Can you work these out from the model? Positions are in its coordinate system, mm. Face numbers are marked on the shaded views. Give positions to 0.01 mm unless a question says otherwise; leave off trailing zeros. Loops run counter-clockwise (first coordinate to the right, second up) from the corner with the lowest first, then second, coordinate; pieces in that order, holes last. Notation, with made-up numbers: M 26,55.5 L 78,55.5 A15 ccw 78,68.5 Z; hole C 70,-33.75 d1. An arc over 180 degrees is marked long. One line per item, written item: value. Start each with the question number.
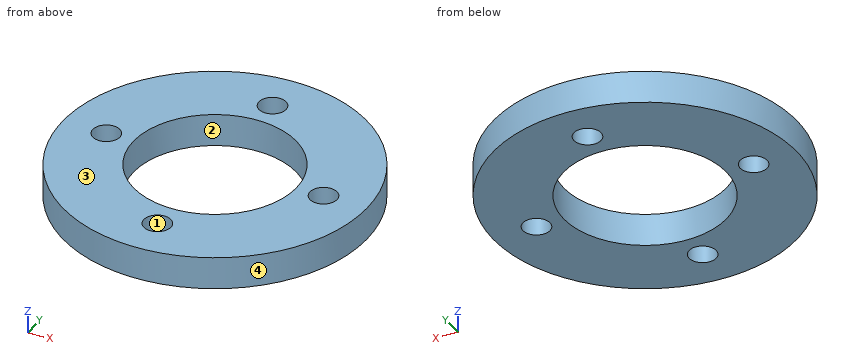
from build123d import *

# Parameters (mm, degrees)
SKETCH_1_R          = 14
EXTRUDE_1_DEPTH     = 3
SKETCH_3_R          = 1.25
CUT_EXTRUDE_1_DEPTH = 3
SKETCH_7_R          = 7.5
CUT_EXTRUDE_2_DEPTH = 10


with BuildPart() as part:
    # 草图1 → 凸台-拉伸1 (new body)
    with BuildSketch(Plane.XY):
        Circle(SKETCH_1_R)
    extrude(amount=EXTRUDE_1_DEPTH)

    # 草图3 → 切除-拉伸1 (cut)
    with BuildSketch(Plane.XY.offset(3)):
        with Locations((10, 0)):
            Circle(SKETCH_3_R)
        with Locations((0, 10)):
            Circle(SKETCH_3_R)
        with Locations((-10, 0)):
            Circle(SKETCH_3_R)
        with Locations((0, -10)):
            Circle(SKETCH_3_R)
    extrude(amount=-CUT_EXTRUDE_1_DEPTH, mode=Mode.SUBTRACT)

    # 草图7 → 切除-拉伸2 (cut)
    with BuildSketch(Plane.XY.offset(3)):
        Circle(SKETCH_7_R)
    extrude(amount=-CUT_EXTRUDE_2_DEPTH, mode=Mode.SUBTRACT)


solid = part.part
Q1. If we section it at A-A, the plane y = 0: Write out the boundary of the cut face in (x, z).
Q2. If we section it at C-C, the plane z = 2: Write out the boundary of the cut face in (x, y).
Q3. If we section it at D-D, the plane y = -5: Write out the boundary of the cut face in (x, z), plus the area to 3 significant figures.
Q4. I need wall thicknesses on line 1 along Y through (x, z) = (0, 2.1); line 2 along X through (y, z) = (0.5, 0.5); line 3 along X through (y, z) = (2, 2.85). Which ranges of each line are inside material? Lowest first, please.
Q5. If we mould it in two halves opening along X, with no side actions, what happens to the marked faces 1, 2, 3 and 4? For each: released by +X, released by -X, zero draft, split by the parting line, or undercut.
Response:
1. outline: M -14,0 L -11.25,0 L -11.25,3 L -14,3 Z; M -8.75,0 L -7.5,0 L -7.5,3 L -8.75,3 Z; M 7.5,0 L 8.75,0 L 8.75,3 L 7.5,3 Z; M 11.25,0 L 14,0 L 14,3 L 11.25,3 Z
2. outline: C 0,0 d28; hole C -10,0 d2.5; hole C 0,0 d15; hole C 0,-10 d2.5; hole C 0,10 d2.5; hole C 10,0 d2.5
3. outline: M -13.08,0 L -5.59,0 L -5.59,3 L -13.08,3 Z; M 5.59,0 L 13.08,0 L 13.08,3 L 5.59,3 Z
3. area: 44.9 mm^2
4. line 1: -14 to -11.25, -8.75 to -7.5, 7.5 to 8.75, 11.25 to 14
4. line 2: -13.99 to -11.15, -8.85 to -7.48, 7.48 to 8.85, 11.15 to 13.99
4. line 3: -13.86 to -7.23, 7.23 to 13.86
5. face 1: undercut
5. face 2: undercut
5. face 3: zero draft
5. face 4: split by the parting line
